```python
from build123d import *

# Parameters (mm, degrees)
F0_R      = 12.5
F1_ANGLE  = -180
F1_FACE_R = 12.5
F2_DEPTH  = 60
F3_R      = 12.5
F4_ANGLE  = 180


with BuildPart() as f1:
    # F0 (on Front) → F1 (revolve)
    with BuildSketch(Plane.XZ):
        with Locations((30, 0)):
            Circle(F0_R)
    revolve(axis=Axis((0, 0, -0.948295), (0, 0, -1)), revolution_arc=F1_ANGLE)

    # F1_face (on face) → F2 (join)
    with BuildSketch(Plane(origin=(30, 0, 0), x_dir=(1, 0, 0), z_dir=(0, -1, 0))):
        Circle(F1_FACE_R)
        with Locations((-60, 0)):
            Circle(F1_FACE_R)
    extrude(amount=F2_DEPTH)

    # F3 (on face) → F4 (revolve)
    with BuildSketch(Plane.XZ.offset(60)):
        with Locations((30, 0)):
            Circle(F3_R)
    revolve(axis=Axis((0, -60, -8.781475), (0, 0, -1)), revolution_arc=F4_ANGLE)


solid = f1.part
```
CAD build for the part. Positions are in the model's coordinates, mm. Coordinates: 2 decimals unless noted, no trailing zeros. Write each loop counter-clockwise with the first axis right and the second up, starting at its lowest first coordinate (ties: lowest second). Pieces come first, ordered by that corner, then holes.
(1) Cut at A-A, the plane z = 0. List the corners of the cut face in (x, y).
(2) Cut at B-B, the plane y = -10.5. List the corners of the cut face in (x, z).
(3) Flat gauge pins, fed straight in: pin 1 (8 mm diameter, centred on x = -8.5, z = -9.5, fed in from -Y); pin 2 (12 mm diameter, centred on x = 13, y = -55.5, fed in from +Z); pin 3 (3 mm diameter, centred on x = 4.5, z = -1, fed in from -Y). Where does each tip first touch, or does it go through?
(4) Cut at C-C, the plane z = -8.75. List the corners of the cut face in (x, y).
(5) Drill centre lines: probe 1 along X at (y, z) = (15, -8.5); probe 2 along X at (y, z) = (-71, 7.25); probe 3 along Y at (x, z) = (-12, -0.25). Where is each one in solid material? Low to high.
Geometry says:
1. outline: (-42.5, -60) arc R42.5 ccw to (42.5, -60) - (42.5, 0) arc R42.5 ccw to (-42.5, 0) - close; hole (-17.5, -60) arc R17.5 ccw to (17.5, -60) - (17.5, 0) arc R17.5 ccw to (-17.5, 0) - close
2. outline: circle Ø25 at (-30, 0); circle Ø25 at (30, 0)
3. pin 1: stops at y = -100.48
3. pin 2: stops at z = 5.94
3. pin 3: stops at y = -102.38
4. outline: (-38.93, -60) arc R38.93 ccw to (38.93, -60) - (38.93, 0) arc R38.93 ccw to (-38.93, 0) - close; hole (-21.07, -60) arc R21.07 ccw to (21.07, -60) - (21.07, 0) arc R21.07 ccw to (-21.07, 0) - close
5. probe 1: x = -36.18 to -14.46, 14.46 to 36.18
5. probe 2: x = -38.65 to -16.48, 16.48 to 38.65
5. probe 3: y = -100.77 to -72.74, 12.74 to 40.77
